from build123d import *

# Parameters (mm, degrees)
SKETCH1_R              = 22.5
SKETCH1_R_2            = 16.9
BOSS_EXTRUDE1_DEPTH    = 19
BOSS_EXTRUDE1_2_DEPTH  = 19
BOSS_EXTRUDE2_DEPTH    = 9
BOSS_EXTRUDE3_DEPTH    = 9
FILLET1_RADIUS         = 9
FILLET1_LENGTH         = 30
FILLET2_RADIUS         = 9
FILLET2_LENGTH         = 30
BOSS_EXTRUDE4_DEPTH    = 5
FILLET3_R              = 1
M10X1_5_TAPPED_HOLE1_D = 9


with BuildPart() as part:
    # Sketch1 → Boss-Extrude1 (new, symmetric)
    with BuildSketch(Plane.XY):
        with Locations((0, 201.2)):
            Circle(SKETCH1_R)
        with Locations((0, 201.2)):
            Circle(SKETCH1_R_2, mode=Mode.SUBTRACT)
    extrude(amount=BOSS_EXTRUDE1_DEPTH, both=True)



with BuildPart() as body_2:
    # Sketch1 → Boss-Extrude1 2 (new, symmetric)
    with BuildSketch(Plane.XY):
        with BuildLine():
            ThreePointArc((30.048695698, 19.826141501), (25.487028558, 25.424621439), (19.899748742, 30))
            ThreePointArc((19.899748742, 30), (0, 36), (-19.899748742, 30))
            ThreePointArc((-19.899748742, 30), (-25.487028558, 25.424621439), (-30.048695698, 19.826141501))
            ThreePointArc((-30.048695698, 19.826141501), (-34.480088784, 10.350047219), (-36, 0))
            Line((-36, 0), (-27, 0))
            ThreePointArc((-27, 0), (0, 27), (27, 0))
            Line((27, 0), (36, 0))
            ThreePointArc((36, 0), (34.480088784, 10.350047219), (30.048695698, 19.826141501))
        make_face()
    extrude(amount=BOSS_EXTRUDE1_2_DEPTH, both=True)


with BuildPart() as part_1:
    add(part.part)

    add(body_2.part)  # Boss-Extrude2 merges body 2
    # Sketch1<3> → Boss-Extrude2 (add, symmetric)
    with BuildSketch(Plane.XY):
        with BuildLine():
            Line((23.655259549, 37.674049083), (10, 167.595165145))
            ThreePointArc((10, 167.595165145), (11.1018188, 177.270143397), (16.188371323, 185.573527784))
            ThreePointArc((16.188371323, 185.573527784), (0, 178.7), (-16.188371323, 185.573527784))
            ThreePointArc((-16.188371323, 185.573527784), (-11.1018188, 177.270143397), (-10, 167.595165145))
            Line((-10, 167.595165145), (-23.655259549, 37.674049083))
            ThreePointArc((-23.655259549, 37.674049083), (-24.2559556, 33.798295304), (-25.233327526, 30))
            Line((-25.233327526, 30), (-19.899748742, 30))
            ThreePointArc((-19.899748742, 30), (0, 36), (19.899748742, 30))
            Line((19.899748742, 30), (25.233327526, 30))
            ThreePointArc((25.233327526, 30), (24.2559556, 33.798295304), (23.655259549, 37.674049083))
        make_face()
        with BuildLine():
            ThreePointArc((-8, 151.2), (0, 159.2), (8, 151.2))
            Line((8, 151.2), (8, 61.2))
            ThreePointArc((8, 61.2), (0, 53.2), (-8, 61.2))
            Line((-8, 61.2), (-8, 151.2))
        make_face(mode=Mode.SUBTRACT)
    extrude(amount=BOSS_EXTRUDE2_DEPTH, both=True)

    # Sketch1<4> → Boss-Extrude3 (add, symmetric)
    with BuildSketch(Plane.XY):
        with BuildLine():
            Line((47, 30), (25.233327526, 30))
            ThreePointArc((25.233327526, 30), (27.281360664, 24.742845095), (30.048695698, 19.826141501))
            ThreePointArc((30.048695698, 19.826141501), (34.480088784, 10.350047219), (36, 0))
            Line((36, 0), (47, 0))
            Line((47, 0), (47, 30))
        make_face()
        with BuildLine():
            ThreePointArc((30.048695698, 19.826141501), (27.281360664, 24.742845095), (25.233327526, 30))
            Line((25.233327526, 30), (19.899748742, 30))
            ThreePointArc((19.899748742, 30), (25.487028558, 25.424621439), (30.048695698, 19.826141501))
        make_face()
        with BuildLine():
            ThreePointArc((-30.048695698, 19.826141501), (-25.487028558, 25.424621439), (-19.899748742, 30))
            Line((-19.899748742, 30), (-25.233327526, 30))
            ThreePointArc((-25.233327526, 30), (-27.281360664, 24.742845095), (-30.048695698, 19.826141501))
        make_face()
        with BuildLine():
            ThreePointArc((-30.048695698, 19.826141501), (-27.281360664, 24.742845095), (-25.233327526, 30))
            Line((-25.233327526, 30), (-47, 30))
            Line((-47, 30), (-47, 0))
            Line((-47, 0), (-36, 0))
            ThreePointArc((-36, 0), (-34.480088784, 10.350047219), (-30.048695698, 19.826141501))
        make_face()
    extrude(amount=BOSS_EXTRUDE3_DEPTH, both=True)

    # Fillet1: full round fillet: the end face becomes a half cylinder, R = half its width
    fillet1_face = Plane((-47, 15, 0), x_dir=(0, 1, 0), z_dir=(-1, 0, 0))  # on the end face: x along it, z out of the body
    fillet1_slab = fillet1_face.offset(-FILLET1_RADIUS / 2) * Box(FILLET1_LENGTH, 2 * FILLET1_RADIUS, FILLET1_RADIUS, mode=Mode.PRIVATE)  # the body's end, R deep
    fillet1_round = Plane((-38, 15, 0), x_dir=(-1, 0, 0), z_dir=(0, 1, 0)) * Cylinder(FILLET1_RADIUS, FILLET1_LENGTH, mode=Mode.PRIVATE)  # its axis R under the face
    add(fillet1_slab - fillet1_round, mode=Mode.SUBTRACT)

    # Fillet2: full round fillet: the end face becomes a half cylinder, R = half its width
    fillet2_face = Plane((47, 15, 0), x_dir=(0, 1, 0), z_dir=(1, 0, 0))  # on the end face: x along it, z out of the body
    fillet2_slab = fillet2_face.offset(-FILLET2_RADIUS / 2) * Box(FILLET2_LENGTH, 2 * FILLET2_RADIUS, FILLET2_RADIUS, mode=Mode.PRIVATE)  # the body's end, R deep
    fillet2_round = Plane((38, 15, 0), x_dir=(1, 0, 0), z_dir=(0, 1, 0)) * Cylinder(FILLET2_RADIUS, FILLET2_LENGTH, mode=Mode.PRIVATE)  # its axis R under the face
    add(fillet2_slab - fillet2_round, mode=Mode.SUBTRACT)

    # Sketch1<5> → Boss-Extrude4 (add, symmetric)
    with BuildSketch(Plane.XY):
        with BuildLine():
            Line((-8, 151.2), (-8, 61.2))
            ThreePointArc((-8, 61.2), (0, 53.2), (8, 61.2))
            Line((8, 61.2), (8, 151.2))
            ThreePointArc((8, 151.2), (0, 159.2), (-8, 151.2))
        make_face()
    extrude(amount=BOSS_EXTRUDE4_DEPTH, both=True)

    # Fillet3
    fillet3_edges = [part_1.edges().sort_by_distance(p)[0] for p in [
        (0, 53.2, 9),
        (-8, 106.2, 9),
        (0, 159.2, 9),
        (8, 106.2, -9),
        (8, 106.2, 9),
        (0, 53.2, -9),
        (0, 159.2, -9),
        (-8, 106.2, -9),
    ]]
    fillet(fillet3_edges, radius=FILLET3_R)

    # M10x1.5 Tapped Hole1 (through all)
    with Locations(Plane(origin=(0, 0, 0), x_dir=(-1, 0, 0), z_dir=(0, -1, 0))):
        with Locations((-38, 0), (38, 0)):
            Hole(M10X1_5_TAPPED_HOLE1_D / 2)


solid = part_1.part
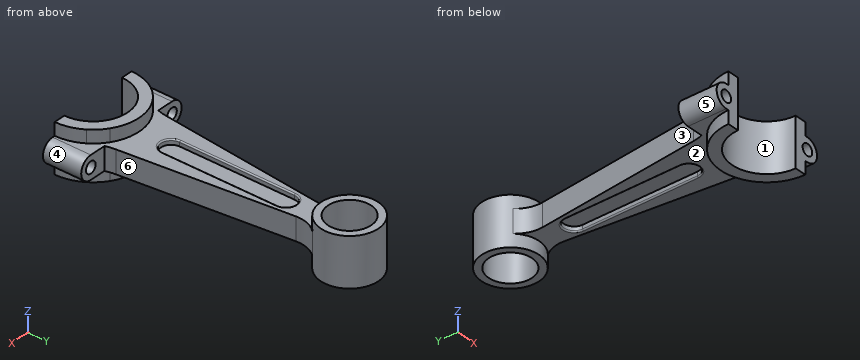
Model file for the job. Use its own axes, mm. Face numbers are marked on the shaded views. A direction names the side the tool comes from. Round coordinates to 2 decimals unless told otherwise and drop trailing zeros. Loops run counter-clockwise (first coordinate to the right, second up) from the corner with the lowest first, then second, coordinate; pieces in that order, holes last. Notation, with made-up numbers: (81.5, 59) -> (94.5, 59) arc R31 ccw to (94.5, 97) -> close; hole circle Ø11 at (8, 34). An arc over 180 degrees is marked (long way). Answer as CSV lines item,"result". Start each with the question number.
1) Mould opens along Y. For the marked faces 1, 2, 3 and 4 say: +Y half, -Y half, draft (parallel to the pull), parting line (faces both ways), or undercut.
2) Slice it at C-C (z = 0). List the corners of the cut face in (x, y), plus the area to 3 significant figures.
3) Pin check, flat tips, straight feed: P1, Ø11.5, axis at x = -38, z = 0, coming from the +Y side; P2, Ø3, axis at x = 20.5, z = -9.5, coming from the +Y side; P3, Ø17.5, axis at x = -0.5, y = 105, coming from the +Z side; P4, Ø8, axis at x = 38, z = 0, coming from the +Y side. Stop position of each tip, or through.
4) Tool access for the marked faces 5 and 6: list every direction of +Z, -Z, +X, -X, +Y, -Y with a clear straight run to the whole face (end or side of a thin tool).
5) Probe line 1 along Z through (x, y) = (-38, 13); line 2 along X through (y, z) = (201, -11); line 3 along Y through (x, z) = (7, -11). List the from-to ranges inside material, lowest first.
6) Slice it at A-A (z = -13). List the corners of the cut face in (x, y), plus the area to 3 significant figures.
7) Slice it at D-D (x = 0). List the corners of the cut face in (y, z), plus the area to 3 significant figures.
8) Slice it at B-B (y = 201.2). List the corners of the cut face in (x, z), plus the area to 3 significant figures.
Filled in:
1,face 1,"-Y half"
1,face 2,"undercut"
1,face 3,"undercut"
1,face 4,"draft"
2,outline,"(-47, 0) -> (-42.5, 0) -> (-42.5, 30) -> (-47, 30) -> close; (-33.5, 0) -> (-27, 0) arc R27 cw to (27, 0) -> (33.5, 0) -> (33.5, 30) -> (25.23, 30) arc R40 cw to (23.66, 37.67) -> (10, 167.6) arc R22.5 cw to (16.19, 185.57) arc R22.5 ccw (long way) to (-16.19, 185.57) arc R22.5 cw to (-10, 167.6) -> (-23.66, 37.67) arc R40 cw to (-25.23, 30) -> (-33.5, 30) -> close; (42.5, 0) -> (47, 0) -> (47, 30) -> (42.5, 30) -> close; hole circle Ø33.8 at (0, 201.2)"
2,area,"6,840 mm2"
3,P1,"stops at y = 30"
3,P2,"stops at y = 213.25"
3,P3,"stops at z = 9"
3,P4,"passes through"
4,face 5,"-X, +Y, -Y"
4,face 6,"+Z, -Z, +X"
5,line 1,"z = -9 to -4.5, 4.5 to 9"
5,line 2,"x = -22.5 to -16.9, 16.9 to 22.5"
5,line 3,"y = 26.08 to 35.31, 179.82 to 185.82, 216.58 to 222.58"
6,outline,"(-36, 0) -> (-27, 0) arc R27 cw to (27, 0) -> (36, 0) arc R36 ccw to start; circle Ø45 at (0, 201.2); hole circle Ø33.8 at (0, 201.2)"
6,area,"1,580 mm2"
7,outline,"(27, -19) -> (36, -19) -> (36, -9) -> (52.2, -9) arc R1 ccw to (53.2, -8) -> (53.2, -5) -> (159.2, -5) -> (159.2, -8) arc R1 ccw to (160.2, -9) -> (178.7, -9) -> (178.7, -19) -> (184.3, -19) -> (184.3, 19) -> (178.7, 19) -> (178.7, 9) -> (160.2, 9) arc R1 ccw to (159.2, 8) -> (159.2, 5) -> (53.2, 5) -> (53.2, 8) arc R1 ccw to (52.2, 9) -> (36, 9) -> (36, 19) -> (27, 19) -> close; (218.1, -19) -> (223.7, -19) -> (223.7, 19) -> (218.1, 19) -> close"
7,area,"2,490 mm2"
8,outline,"(-22.5, -19) -> (-16.9, -19) -> (-16.9, 19) -> (-22.5, 19) -> close; (16.9, -19) -> (22.5, -19) -> (22.5, 19) -> (16.9, 19) -> close"
8,area,"426 mm2"
